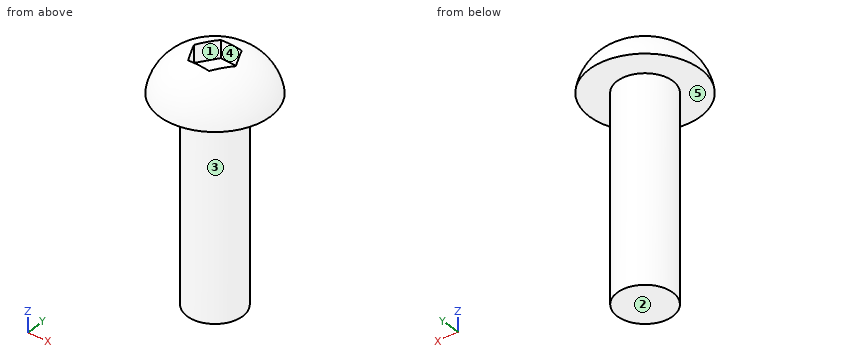
```python
from build123d import *

# Parameters (mm, degrees)
F0_R     = 3
F0_R_2   = 1.5
F1_DEPTH = 2
F2_DEPTH = 11
F6_DEPTH = 1.5


# Not quite as in the source:
# - a fillet or chamfer that OpenCascade refuses, or shapes differently, is made with other operations: its cross-section is extruded or revolved along the edge and cut away or added


with BuildPart() as f1:
    # F0 (on Top) → F1 (new body)
    with BuildSketch(Plane.XY):
        Circle(F0_R)
        Circle(F0_R_2, mode=Mode.SUBTRACT)
        Circle(F0_R_2)
    extrude(amount=F1_DEPTH)

    # F0 (on Top) → F2 (join)
    with BuildSketch(Plane.XY):
        Circle(F0_R_2)
    extrude(amount=-F2_DEPTH)

    # F3: fillet of radius 2.3417871555 on 1 edges, made by hand

    # F3_s1 → F3_t2 (revolve, cut)
    with BuildSketch(Plane.XZ):
        with BuildLine():
            ThreePointArc((3, 0), (2.2135791593, 1.4308323542), (0.6832892667, 2))
            Line((0.6832892667, 2), (3, 2))
            Line((3, 2), (3, 0))
        make_face()
    revolve(axis=Axis((0, 0, 2), (0, 0, 1)), mode=Mode.SUBTRACT)

    # F5 (on offset) → F6 (cut)
    with BuildSketch(Plane.XY.offset(2.5)):
        Polygon((0.5268892093, -1.0919650915), (1.209114114, -0.0896831055), (0.6822249046, 1.002281986), (-0.5268892093, 1.0919650915), (-1.209114114, 0.0896831055), (-0.6822249046, -1.002281986), align=None)
    extrude(amount=-F6_DEPTH, mode=Mode.SUBTRACT)


solid = f1.part
```
Part model, mm, in its own coordinate system. Face numbers are marked on the shaded views. A direction names the side the tool comes from. Round coordinates to 2 decimals unless told otherwise and drop trailing zeros. Order: outer loops, then holes, each group sorted by start corner. A loop starts at its lowest first (then second) coordinate and runs counter-clockwise, first axis right, second up. Notation, with made-up numbers: M 62,62.25 L 86,62.25 A32 ccw 86,97.25 Z; hole C 85,-14.5 d11. An arc over 180 degrees is marked long. Answer in a Markdown table with one row per item. Add a question column.
Q1. Mould opens along Y. For the marked faces 3, 4 and 5 say: +Y half, -Y half, draft (parallel to the pull), parting line (faces both ways), or undercut.
Q2. 3-axis set-ups, long thin cutter, end or side, ignore diameter. For the marked faces 1 and 2: which of +Z, -Z, +X, -X, +Y, -Y reach the whole face in a straight line?
Q3. Wall check: L1, parallel to Y at x = 0, z = -9.5; L2, parallel to Y at x = 1.25, z = -8.5; L3, parallel to Z at x = -1.5, y = 2. Give the ranges that are in metal, low to high. Write a range as from..to.
Q4. Cut at A-A on z = -5.75. Give the cut face in (x, y).
Q5. Pin check, flat tips, straight feed: pin 1 (1 mm diameter, centred on y = 1.5, z = -5.5, fed in from +X); pin 2 (2 mm diameter, centred on x = -0.5, z = -5.5, fed in from +Y); pin 3 (0.7 mm diameter, centred on x = 0, y = 0, fed in from +Z). Stop position of each tip, or through.
Established:
| question | item | result |
|---|---|---|
| 1 | face 3 | parting line |
| 1 | face 4 | undercut |
| 1 | face 5 | draft |
| 2 | face 1 | +Z |
| 2 | face 2 | -Z, +X, -X, +Y, -Y |
| 3 | L1 | y = -1.5..1.5 |
| 3 | L2 | y = -0.83..0.83 |
| 3 | L3 | z = 0..1.14 |
| 4 | outline | C 0,0 d3 |
| 5 | pin 1 | stops at x = 1.12 |
| 5 | pin 2 | stops at y = 1.5 |
| 5 | pin 3 | stops at z = 1 |
